The listing builds one solid part. Answer for the finished solid, in the listing's coordinates (mm). A direction names the side the tool comes from. Give positions to 0.01 mm unless a question says otherwise; leave off trailing zeros. Write each loop counter-clockwise with the first axis right and the second up, starting at its lowest first coordinate (ties: lowest second). Pieces come first, ordered by that corner, then holes. Notation, with made-up numbers: (-29, -12.75) - (-16, -12.75) arc R18 cw to (-16, -5.75) - close; hole circle Ø8 at (23.25, 79.25). An arc over 180 degrees is marked (long way). Return JSON: item names as keys, results as strings.
from build123d import *

# Parameters (mm, degrees)
SKETCH1_W           = 103
SKETCH1_H           = 103
BOSS_EXTRUDE1_DEPTH = 104
SKETCH2_R           = 5
BOSS_EXTRUDE2_DEPTH = 15
BOSS_EXTRUDE3_START = 15
SKETCH3_R           = 5
BOSS_EXTRUDE3_DEPTH = 15
SKETCH4_R           = 17.5
SKETCH4_R_2         = 12.5
CUT_EXTRUDE1_DEPTH  = 20


with BuildPart() as part:
    # Sketch1 → Boss-Extrude1 (new body)
    with BuildSketch(Plane(origin=(0, 0, 0), x_dir=(1, 0, 0), z_dir=(0, 1, 0))):
        Rectangle(SKETCH1_W, SKETCH1_H)
    extrude(amount=BOSS_EXTRUDE1_DEPTH)

    # Sketch2 → Boss-Extrude2 (add)
    with BuildSketch(Plane.XY.offset(51.5)):
        with Locations(Location((-0.5, 51.997596098, 0), (0, 0, 180))):
            Circle(SKETCH2_R)
    extrude(amount=BOSS_EXTRUDE2_DEPTH)

    # Sketch3 → Boss-Extrude3 (add)
    with BuildSketch(Plane(origin=(0, 0, -51.5), x_dir=(-1, 0, 0), z_dir=(0, 0, -1)).offset(BOSS_EXTRUDE3_START)):
        with Locations((0.5, 51.997596098)):
            Circle(SKETCH3_R)
    extrude(amount=-BOSS_EXTRUDE3_DEPTH)

    # Sketch4 → Cut-Extrude1 (cut)
    with BuildSketch(Plane.ZY.offset(51.5)):
        with Locations((0, 52)):
            Circle(SKETCH4_R)
        with Locations((0, 52)):
            Circle(SKETCH4_R_2, mode=Mode.SUBTRACT)
    extrude(amount=-CUT_EXTRUDE1_DEPTH, mode=Mode.SUBTRACT)


solid = part.part
Item 1: Flat-ended cylindrical pins translate along their axes: P1, Ø2, axis at x = 1.5, y = 88.5, coming from the -Z side; P2, Ø10, axis at x = 29.5, y = 84.5, coming from the +Z side. Find the tip coordinate at first contact, or state that the pin passes through.
Answer below:
{"P1": "stops at z = -51.5", "P2": "stops at z = 51.5"}
Item 2: A cutting plane is placed at A-A on z = 0. Determine the outline of the cut face in (x, y), then the cut area to 3 significant figures.
Answer below:
{"outline": "(-51.5, 0) - (51.5, 0) - (51.5, 104) - (-51.5, 104) - (-51.5, 69.5) - (-31.5, 69.5) - (-31.5, 64.5) - (-51.5, 64.5) - (-51.5, 39.5) - (-31.5, 39.5) - (-31.5, 34.5) - (-51.5, 34.5) - close", "area": "10,500 mm²"}
Item 3: For faces 4 (the face through (-3.188, 47.782, 58.895)), 5 (the face through (-31.5, 41, 8)), 6 (the face through (0.584, 47.116, -59.105)), 7 (the face through (0, 52, 66.5)), 8 (the face through (-51.5, 52, 0)), determine the directions among +Z, -Z, +X, -X, +Y, -Y from which every point of the face is accessible in a straight line to the end or side of a thin tool.
Answer below:
{"face 4": "+Z", "face 5": "-X", "face 6": "-Z", "face 7": "+Z, +X, -X, +Y, -Y", "face 8": "+Z, -Z, -X, +Y, -Y"}
Item 4: A cutting plane is placed at B-B on x = -0.5. Determine the outline of the cut face in (y, z), then the cut area to 3 significant figures.
Answer below:
{"outline": "(0, -51.5) - (47, -51.5) - (47, -66.5) - (57, -66.5) - (57, -51.5) - (104, -51.5) - (104, 51.5) - (57, 51.5) - (57, 66.5) - (47, 66.5) - (47, 51.5) - (0, 51.5) - close", "area": "11,000 mm²"}
Item 5: Consider L1, parallel to Y at x = -40, z = 0; L2, parallel to Z at x = 26, y = 100.5. Determine where each line is inside the solid, lowest interval first.
Answer below:
{"L1": "y = 0 to 34.5, 39.5 to 64.5, 69.5 to 104", "L2": "z = -51.5 to 51.5"}
Item 6: A cutting plane is placed at D-D on x = 14.5. Determine the outline of the cut face in (y, z).
Answer below:
{"outline": "(0, -51.5) - (104, -51.5) - (104, 51.5) - (0, 51.5) - close"}
Item 7: A cutting plane is placed at C-C on y = 76. Determine the outline of the cut face in (x, z).
Answer below:
{"outline": "(-51.5, -51.5) - (51.5, -51.5) - (51.5, 51.5) - (-51.5, 51.5) - close"}
Item 8: The mould has two halves that part along Z. Classify faces 1 (the face through (-12, 51, -51.5)), 2 (the face through (-51.5, 51, -22)), 3 (the face through (-41.64, 64.394, -1.627)): +Z half, -Z half, draft (parallel to the pull), parting line (faces both ways), or undercut.
Answer below:
{"face 1": "-Z half", "face 2": "draft", "face 3": "undercut"}
